Job drawing, mm, ordinate dimensions from the low corner. One solid piece. A direction names the side the tool comes from. Round coordinates to 2 decimals unless told otherwise and drop trailing zeros. Write each loop counter-clockwise with the first axis right and the second up, starting at its lowest first coordinate (ties: lowest second). Pieces come first, ordered by that corner, then holes. Notation, with made-up numbers: M 75,-40 L 122,-40 A27 ccw 122,-19 Z; hole C 24.25,75.25 d3. An arc over 180 degrees is marked long. Answer as a JSON object with one key per item and string values. Group by question number.
1. Drill centre lines: line 1 (Z direction, x = 35, y = 39); line 2 (Y direction, x = 56, z = 55) (1 decimal); line 3 (X direction, y = 109, z = 87.5) (1 decimal). Where is each one in solid material? Low to high. Write a range as from..to.
2. Two-plate mould, pull along X, no slides. Class the marked faces 4, 5 and 6: +X half, -X half, draft (parallel to the pull), parting line (faces both ways), or undercut.
3. Which spindle directions (+Z, -Z, +X, -X, +Y, -Y) get a long thin tool onto all of the face, cutting with end or side? Do the marked faces 1, 2 and 3. Say none if no direction does.
4. Band-saw the part on D-D, the plane x = 10. Write the cut outline in (y, z) (1 decimal).
5. Band-saw the part on A-A, the plane z = 117. Write the cut outline in (x, y) (1 decimal), plus the area to 4 significant figures.
6. Drop flat-ended pins along their axis: pin 1 (24 mm diameter, centred on x = 75, z = 17, fed in from +Y); pin 2 (2 mm diameter, centred on x = 17.5, z = 98.5, fed in from -Y) (1 decimal); pin 3 (5 mm diameter, centred on x = 34, y = 28.5, fed in from +Z). Give the stop position or say it passes through.
7. Band-saw the part on B-B, the plane x = 76. Write the cut outline in (y, z) (1 decimal), plus the area to 3 significant figures.
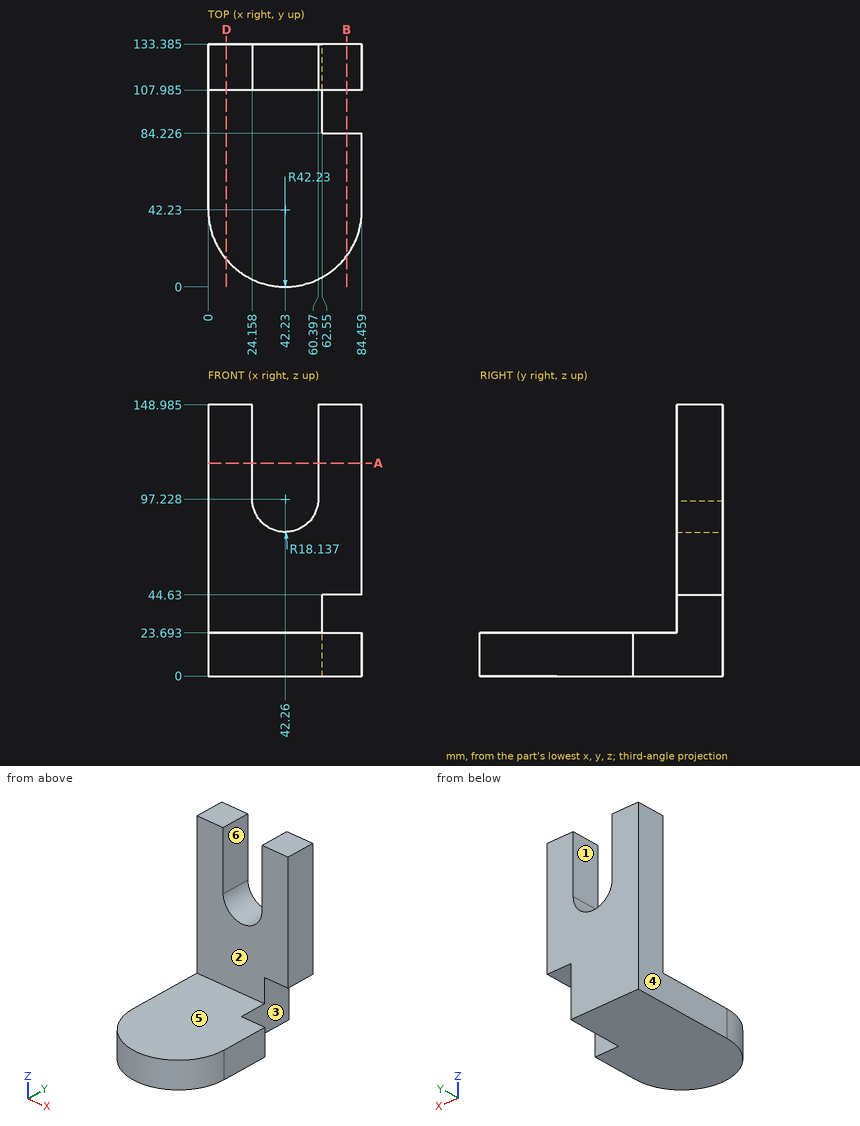
Worked answers:
{
 "1": {"line 1": "z = 0..23.69", "line 2": "y = 108..133.4", "line 3": "x = 0..27, 57.6..84.5"},
 "2": {"face 4": "-X half", "face 5": "draft", "face 6": "undercut"},
 "3": {"face 1": "+Z, +Y, -Y", "face 2": "+Z, +X, -X, -Y", "face 3": "-Z, +X, +Y"},
 "4": {"outline": "M 14.9,0 L 133.4,0 L 133.4,149 L 108,149 L 108,23.7 L 14.9,23.7 Z"},
 "5": {"outline": "M 0,108 L 24.2,108 L 24.2,133.4 L 0,133.4 Z; M 60.4,108 L 84.5,108 L 84.5,133.4 L 60.4,133.4 Z", "area": "1,225 mm^2"},
 "6": {"pin 1": "stops at y = 84.23", "pin 2": "stops at y = 108", "pin 3": "stops at z = 23.69"},
 "7": {"outline": "M 16.9,0 L 84.2,0 L 84.2,23.7 L 16.9,23.7 Z; M 108,44.6 L 133.4,44.6 L 133.4,149 L 108,149 Z", "area": "4,250 mm^2"}
}
